The model under review builds one solid part; all positions refer to its coordinate system, in mm. Face numbers are marked on the shaded views. Coordinates: 2 decimals unless noted, no trailing zeros. Loops run counter-clockwise (first coordinate to the right, second up) from the corner with the lowest first, then second, coordinate; pieces in that order, holes last. Notation, with made-up numbers: M -37.5,53 L -18.5,53 A25 cw -18.5,79 Z; hole C 74,-16 d7. An arc over 180 degrees is marked long. One line per item, written item: value.
```python
from build123d import *

# Parameters (mm, degrees)
SKETCH1_R           = 7.3
BOSS_EXTRUDE1_DEPTH = 30
SKETCH2_R           = 6.5
CUT_EXTRUDE1_DEPTH  = 6
SKETCH3_OUTSIDE_W   = 23.884
SKETCH3_OUTSIDE_H   = 23.884
CUT_EXTRUDE3_DEPTH  = 22
FILLET2_R           = 0.5


with BuildPart() as part:
    # Sketch1 → Boss-Extrude1 (new body)
    with BuildSketch(Plane.XY):
        Circle(SKETCH1_R)
    extrude(amount=BOSS_EXTRUDE1_DEPTH)

    # Sketch2 → Cut-Extrude1 (cut)
    with BuildSketch(Plane.XY.offset(30)):
        Circle(SKETCH2_R)
    extrude(amount=-CUT_EXTRUDE1_DEPTH, mode=Mode.SUBTRACT)

    # Sketch3 outside → Cut-Extrude3 (cut)
    with BuildSketch(Plane(origin=(0, 0, 0), x_dir=(-1, 0, 0), z_dir=(0, 0, -1))):
        Rectangle(SKETCH3_OUTSIDE_W, SKETCH3_OUTSIDE_H)
        Polygon((7.3, 0), (5.161879503, 5.161879503), (0, 7.3), (-5.161879503, 5.161879503), (-7.3, 0), (-5.161879503, -5.161879503), (0, -7.3), (5.161879503, -5.161879503), align=None, mode=Mode.SUBTRACT)
    extrude(amount=-CUT_EXTRUDE3_DEPTH, mode=Mode.SUBTRACT)

    # Fillet2
    # the kernel refuses this fillet: 0.5 mm, written as the material it takes off along each edge
    with BuildSketch(Plane(origin=(0, 0, 22), x_dir=(1, 0, 0), z_dir=(0, 1, 0))) as fillet2_piece_1_section:
        with BuildLine():
            CenterArc((7.3 - FILLET2_R, -FILLET2_R), FILLET2_R, 0, 90)
            Line((7.3, -FILLET2_R), (7.3, 0))
            Line((7.3, 0), (7.3 - FILLET2_R, 0))
        make_face()
    fillet2_piece_1 = revolve(axis=Axis((0, 0, 22), (0, 0, -1)), revolution_arc=45, mode=Mode.PRIVATE)
    fillet2_piece_1 = split(fillet2_piece_1, bisect_by=Plane(origin=(6.230939751, -2.580939751, 22.141608604), z_dir=(0.9238795325112824, -0.3826834323651005, 0)), keep=Keep.TOP, mode=Mode.PRIVATE)
    add(fillet2_piece_1, mode=Mode.SUBTRACT)
    with BuildSketch(Plane(origin=(0, 0, 22), x_dir=(0.7071067811865394, -0.7071067811865557, 0), z_dir=(0.7071067811865557, 0.7071067811865394, 0))) as fillet2_piece_2_section:
        with BuildLine():
            CenterArc((7.3 - FILLET2_R, -FILLET2_R), FILLET2_R, 0, 90)
            Line((7.3 - FILLET2_R, 0), (7.3, 0))
            Line((7.3, 0), (7.3, -FILLET2_R))
        make_face()
    fillet2_piece_2 = revolve(axis=Axis((0, 0, 22), (0, 0, -1)), revolution_arc=45, mode=Mode.PRIVATE)
    fillet2_piece_2 = split(fillet2_piece_2, bisect_by=Plane(origin=(2.580939751, -6.230939751, 22.141608605), z_dir=(0.3826834323650794, -0.9238795325112911, 0)), keep=Keep.TOP, mode=Mode.PRIVATE)
    add(fillet2_piece_2, mode=Mode.SUBTRACT)
    with BuildSketch(Plane(origin=(0, 0, 22), x_dir=(0, -1, 0), z_dir=(1, 0, 0))) as fillet2_piece_3_section:
        with BuildLine():
            CenterArc((7.3 - FILLET2_R, -FILLET2_R), FILLET2_R, 0, 90)
            Line((7.3 - FILLET2_R, 0), (7.3, 0))
            Line((7.3, 0), (7.3, -FILLET2_R))
        make_face()
    fillet2_piece_3 = revolve(axis=Axis((0, 0, 22), (0, 0, -1)), revolution_arc=45, mode=Mode.PRIVATE)
    fillet2_piece_3 = split(fillet2_piece_3, bisect_by=Plane(origin=(-2.580939751, -6.230939751, 22.141608604), z_dir=(-0.38268343236510044, -0.9238795325112824, 0)), keep=Keep.TOP, mode=Mode.PRIVATE)
    add(fillet2_piece_3, mode=Mode.SUBTRACT)
    with BuildSketch(Plane(origin=(0, 0, 22), x_dir=(-0.7071067811865553, -0.7071067811865397, 0), z_dir=(0.7071067811865397, -0.7071067811865553, 0))) as fillet2_piece_4_section:
        with BuildLine():
            CenterArc((7.3 - FILLET2_R, -FILLET2_R), FILLET2_R, 0, 90)
            Line((7.3 - FILLET2_R, 0), (7.3, 0))
            Line((7.3, 0), (7.3, -FILLET2_R))
        make_face()
    fillet2_piece_4 = revolve(axis=Axis((0, 0, 22), (0, 0, -1)), revolution_arc=45, mode=Mode.PRIVATE)
    fillet2_piece_4 = split(fillet2_piece_4, bisect_by=Plane(origin=(-6.230939751, -2.580939751, 22.141608603), z_dir=(-0.9238795325112912, -0.3826834323650791, 0)), keep=Keep.TOP, mode=Mode.PRIVATE)
    add(fillet2_piece_4, mode=Mode.SUBTRACT)
    with BuildSketch(Plane(origin=(0, 0, 22), x_dir=(-1, 0, 0), z_dir=(0, -1, 0))) as fillet2_piece_5_section:
        with BuildLine():
            CenterArc((7.3 - FILLET2_R, -FILLET2_R), FILLET2_R, 0, 90)
            Line((7.3 - FILLET2_R, 0), (7.3, 0))
            Line((7.3, 0), (7.3, -FILLET2_R))
        make_face()
    fillet2_piece_5 = revolve(axis=Axis((0, 0, 22), (0, 0, -1)), revolution_arc=45, mode=Mode.PRIVATE)
    fillet2_piece_5 = split(fillet2_piece_5, bisect_by=Plane(origin=(-6.230939751, 2.580939751, 22.141608604), z_dir=(-0.9238795325112823, 0.38268343236510055, 0)), keep=Keep.TOP, mode=Mode.PRIVATE)
    add(fillet2_piece_5, mode=Mode.SUBTRACT)
    with BuildSketch(Plane(origin=(0, 0, 22), x_dir=(-0.7071067811865395, 0.7071067811865556, 0), z_dir=(-0.7071067811865556, -0.7071067811865395, 0))) as fillet2_piece_6_section:
        with BuildLine():
            CenterArc((7.3 - FILLET2_R, -FILLET2_R), FILLET2_R, 0, 90)
            Line((7.3 - FILLET2_R, 0), (7.3, 0))
            Line((7.3, 0), (7.3, -FILLET2_R))
        make_face()
    fillet2_piece_6 = revolve(axis=Axis((0, 0, 22), (0, 0, -1)), revolution_arc=45, mode=Mode.PRIVATE)
    fillet2_piece_6 = split(fillet2_piece_6, bisect_by=Plane(origin=(-2.580939751, 6.230939751, 22.141608604), z_dir=(-0.3826834323650789, 0.9238795325112913, 0)), keep=Keep.TOP, mode=Mode.PRIVATE)
    add(fillet2_piece_6, mode=Mode.SUBTRACT)
    with BuildSketch(Plane(origin=(0, 0, 22), x_dir=(0, 1, 0), z_dir=(-1, 0, 0))) as fillet2_piece_7_section:
        with BuildLine():
            CenterArc((7.3 - FILLET2_R, -FILLET2_R), FILLET2_R, 0, 90)
            Line((7.3, -FILLET2_R), (7.3, 0))
            Line((7.3, 0), (7.3 - FILLET2_R, 0))
        make_face()
    fillet2_piece_7 = revolve(axis=Axis((0, 0, 22), (0, 0, -1)), revolution_arc=45, mode=Mode.PRIVATE)
    fillet2_piece_7 = split(fillet2_piece_7, bisect_by=Plane(origin=(2.580939751, 6.230939751, 22.141608604), z_dir=(0.38268343236510044, 0.9238795325112824, 0)), keep=Keep.TOP, mode=Mode.PRIVATE)
    add(fillet2_piece_7, mode=Mode.SUBTRACT)
    with BuildSketch(Plane(origin=(0, 0, 22), x_dir=(0.7071067811865556, 0.7071067811865395, 0), z_dir=(-0.7071067811865395, 0.7071067811865556, 0))) as fillet2_piece_8_section:
        with BuildLine():
            CenterArc((7.3 - FILLET2_R, -FILLET2_R), FILLET2_R, 0, 90)
            Line((7.3, -FILLET2_R), (7.3, 0))
            Line((7.3, 0), (7.3 - FILLET2_R, 0))
        make_face()
    fillet2_piece_8 = revolve(axis=Axis((0, 0, 22), (0, 0, -1)), revolution_arc=45, mode=Mode.PRIVATE)
    fillet2_piece_8 = split(fillet2_piece_8, bisect_by=Plane(origin=(6.230939751, 2.580939751, 22.141608603), z_dir=(0.9238795325112913, 0.38268343236507885, 0)), keep=Keep.TOP, mode=Mode.PRIVATE)
    add(fillet2_piece_8, mode=Mode.SUBTRACT)


solid = part.part
```
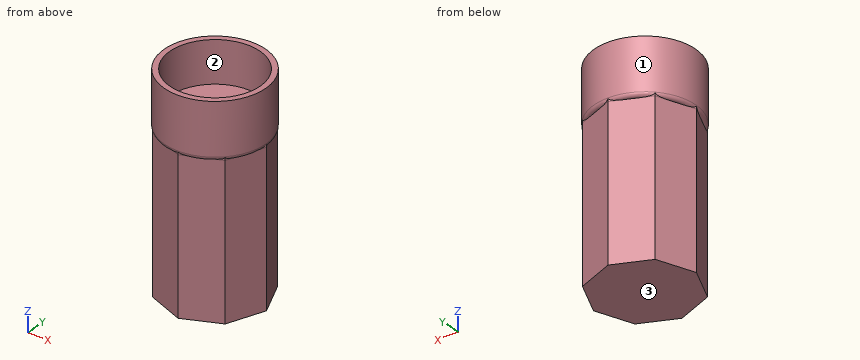
(1) To check wall thickness, follow L1, parallel to Y at x = 0, z = 27.7; L2, parallel to Z at x = -4.75, y = -2.5; L3, parallel to Y at x = -4, z = 24.5. State the ranges of each line that lie inside material, in increasing order. Write a range as [from, to].
Checks:
L1: [-7.3, -6.5], [6.5, 7.3]
L2: [0, 24]
L3: [-6.11, -5.12], [5.12, 6.11]
(2) Draft analysis for pull direction X (two halves, no side actions). For the marked faces 1, 2 and 3, state which applies: pulls with the +X half, pulls with the -X half, needs draft (parallel to the pull), parting line crosses it, or undercut.
Checks:
face 1: parting line crosses it
face 2: undercut
face 3: needs draft
(3) Insertion check: pin 1 Ø4 at (x, y) = (3, -1.5) entering from +Z; pin 2 Ø4 at (y, z) = (3.5, 20) entering from -X; pin 3 Ø2 at (x, z) = (4.5, 14.5) entering from +Y. Each pin has a flat end and moves straight along its axis. Give the tip position at first contact, or say it passes through.
Checks:
pin 1: z = 24
pin 2: x = -6.68
pin 3: y = 5.85
(4) Add section A-A on z = 18.25. State the section outline as (x, y) points, then the cut area to 3 significant figures.
Checks:
outline: M -7.3,0 L -5.16,-5.16 L 0,-7.3 L 5.16,-5.16 L 7.3,0 L 5.16,5.16 L 0,7.3 L -5.16,5.16 Z
area: 151 mm^2
(5) Add section B-B on z = 26. State the section outline as (x, y) points, then the cut area to 3 significant figures.
Checks:
outline: C 0,0 d14.6; hole C 0,0 d13
area: 34.7 mm^2
